Design review of the part built by this model. Coordinates are the model's own, in mm. A direction names the side the tool comes from. Coordinates: 2 decimals unless noted, no trailing zeros. Loops run counter-clockwise (first coordinate to the right, second up) from the corner with the lowest first, then second, coordinate; pieces in that order, holes last.
Q1. Draft analysis for pull direction Y (two halves, no side actions). For faces 4 (the face through (58, -80, 11)), 5 (the face through (30, 11, 16.9)), 6 (the face through (58, -5, 4)), state which applies: released by +Y, released by -Y, zero draft, split by the parting line, or undercut.
Q2. Add section D-D on x = 7. Give the boundary of the cut face in (y, z).
Q3. Machinability: for faces 1 (the face through (56, -42, 11)), 2 (the face through (44, 11, 19)), 3 (the face through (16, 11, 19)), which of the approach directions +Z, -Z, +X, -X, +Y, -Y give a long, thin tool a straight path to every point of the face, cutting with its end or side? Answer none if there is none.
Q4. Wall thickness on probe 1 along Y at (x, z) = (24, 17.95); probe 2 along X at (y, z) = (-59, 15); probe 3 along Y at (x, z) = (36.5, 3.5): over which ranges is each line inside the solid? List them lowest first.
Q5. Add section C-C on y = -22. Give the boundary of the cut face in (x, z).
Q6. Add section B-B on y = 13.6. Give the boundary of the cut face in (x, z), and give its area (3 significant figures).
Q7. Add section A-A on x = 24. Give the boundary of the cut face in (y, z).
Q8. For P1, Ø1.8, axis at x = 24, y = 13.6, coming from the +Z side; P2, Ø14.5, axis at x = 27.5, y = 14, coming from the +Z side; P3, Ø11.5, axis at y = -43, z = 6, coming from the -X side; P4, Ø2.5, axis at y = 13.5, z = 19, coming from the +X side, all flat-tipped, find the tip position at first contact; note any pin that passes through.
```python
from build123d import *

# Parameters (mm, degrees)
SKETCH1_W           = 60
SKETCH1_H           = 23.2
BOSS_EXTRUDE1_DEPTH = 4.4
SKETCH2_W           = 28
SKETCH2_H           = 3.2
BOSS_EXTRUDE2_DEPTH = 13.2
SKETCH3_W           = 4
SKETCH3_H           = 15.2
BOSS_EXTRUDE3_DEPTH = 80
SKETCH4_W           = 4
SKETCH4_H           = 68
BOSS_EXTRUDE4_DEPTH = 4
FILLET1_SIZE        = 5
FILLET2_SIZE        = 4
SKETCH5_R           = 1.5
CUT_EXTRUDE1_DEPTH  = 10


with BuildPart() as part:
    # Sketch1 → Boss-Extrude1 (new body)
    with BuildSketch(Plane(origin=(0, 0, 0), x_dir=(1, 0, 0), z_dir=(0, 1, 0))):
        with Locations((30, -11.6)):
            Rectangle(SKETCH1_W, SKETCH1_H)
    extrude(amount=BOSS_EXTRUDE1_DEPTH)

    # Sketch2 → Boss-Extrude2 (add)
    with BuildSketch(Plane(origin=(0, 4.4, 0), x_dir=(1, 0, 0), z_dir=(0, 1, 0))):
        with Locations((30, -18.5)):
            Rectangle(SKETCH2_W, SKETCH2_H)
    extrude(amount=BOSS_EXTRUDE2_DEPTH)

    # Sketch3 → Boss-Extrude3 (add)
    with BuildSketch(Plane(origin=(0, 0, 0), x_dir=(-1, 0, 0), z_dir=(0, -1, 0))):
        with Locations((-58, -11.6)):
            Rectangle(SKETCH3_W, SKETCH3_H)
    extrude(amount=BOSS_EXTRUDE3_DEPTH)

    # Sketch4 → Boss-Extrude4 (add)
    with BuildSketch(Plane.ZY.offset(-56)):
        with Locations((21.2, -46)):
            Rectangle(SKETCH4_W, SKETCH4_H)
        with Locations((2, -46)):
            Rectangle(SKETCH4_W, SKETCH4_H)
    extrude(amount=-BOSS_EXTRUDE4_DEPTH)

    # Fillet1
    # a fillet whose section is not a circle: 5 mm, written as the material it adds along each edge
    with BuildSketch(Plane(origin=(56, 0, 4), x_dir=(-1, 0, 0), z_dir=(0, 0, 1))) as fillet1_piece_1:
        with BuildLine():
            Bezier((FILLET1_SIZE, 0), (0, 0), (0, FILLET1_SIZE), weights=[1, 0.052631579, 1])
            Line((0, FILLET1_SIZE), (0, 0))
            Line((0, 0), (FILLET1_SIZE, 0))
        make_face()
    extrude(amount=15.2)

    # Fillet2
    # a fillet whose section is not a circle: 4 mm, written as the material it takes off along each edge
    with BuildSketch(Plane(origin=(46, -12, 0), x_dir=(0, 0, 1), z_dir=(1, 0, 0)), Plane(origin=(46, -12, 23.2), x_dir=(0, -1, 0), z_dir=(1, 0, 0))) as fillet2_piece_1:
        with BuildLine():
            Bezier((FILLET2_SIZE, 0), (0, 0), (0, FILLET2_SIZE), weights=[1, 0.052631579, 1])
            Line((0, FILLET2_SIZE), (0, 0))
            Line((0, 0), (FILLET2_SIZE, 0))
        make_face()
    extrude(amount=24, mode=Mode.SUBTRACT)

    # Sketch5 → Cut-Extrude1 (cut)
    with BuildSketch(Plane.XY.offset(20.1)):
        with Locations((24, 13.6)):
            Circle(SKETCH5_R)
    extrude(amount=-CUT_EXTRUDE1_DEPTH, mode=Mode.SUBTRACT)


solid = part.part
```
Entries:
1. face 4: released by -Y
1. face 5: zero draft
1. face 6: undercut
2. outline: (0, 0) - (4.4, 0) - (4.4, 23.2) - (0, 23.2) - close
3. face 1: +Z, -Z, -X, -Y
3. face 2: +Z, -Z, +X, +Y
3. face 3: +Z, -Z, -X, +Y
4. probe 1: y = 0 to 12.1, 15.1 to 17.6
4. probe 2: x = 56 to 60
4. probe 3: y = 0 to 4.4
5. outline: (56, 0) - (60, 0) - (60, 23.2) - (56, 23.2) - close
6. outline: (16, 16.9) - (22.5, 16.9) - (22.5, 20.1) - (16, 20.1) - close; (25.5, 16.9) - (44, 16.9) - (44, 20.1) - (25.5, 20.1) - close
6. area: 80.0 mm2
7. outline: (0, 0) - (4.4, 0) - (4.4, 16.9) - (12.1, 16.9) - (12.1, 20.1) - (4.4, 20.1) - (4.4, 23.2) - (0, 23.2) - close; (15.1, 16.9) - (17.6, 16.9) - (17.6, 20.1) - (15.1, 20.1) - close
8. P1: passes through
8. P2: stops at z = 20.1
8. P3: stops at x = 56
8. P4: stops at x = 44
